Can you work these out from the model? Positions are in its coordinate system, mm. Face numbers are marked on the shaded views. A direction names the side the tool comes from. Coordinates: 2 decimals unless noted, no trailing zeros. Order: outer loops, then holes, each group sorted by start corner. A loop starts at its lowest first (then second) coordinate and runs counter-clockwise, first axis right, second up. Notation, with made-up numbers: M 67.25,86.5 L 90.25,86.5 A24 ccw 90.25,117.5 Z; hole C -40,65.5 d11. An arc over 180 degrees is marked long. Answer as CSV lines item,"result". Start each with the question number.
1. Will these pins go through, and if not, where does the flat tip stop? pin 1 (5 mm diameter, centred on y = -106.5, z = 1257.5, fed in from -X); pin 2 (8 mm diameter, centred on x = 134.5, z = 938.5, fed in from -Y); pin 3 (10 mm diameter, centred on y = -179, z = 1516.5, fed in from +X).
2. If we section it at A-A (x = 239): List the corners of the cut face in (y, z) for me.
3. I need wall thicknesses on line 1 along Z through (x, y) = (267, -102.5); line 2 along X through (y, z) = (-146, 1263.5). Which ranges of each line are inside material? Lowest first, please. Write a range as from..to.
4. If we section it at D-D (z = 1408): List the corners of the cut face in (x, y) for me, plus the area to 3 significant figures.
5. On a 3-axis mill with a long thin cutter (end or side, diameter ignored), from which of +Z, -Z, +X, -X, +Y, -Y can I reach the whole of each face in a straight line? I mean the marked faces 1, 2 and 3. Say none if no direction works.
6. If we section it at B-B (y = 0): List the corners of the cut face in (x, z) for me.
7. If we mould it in two halves opening along Z, with no side actions, what happens to the marked faces 4, 5 and 6? For each: released by +Z, released by -Z, zero draft, split by the parting line, or undercut.
```python
from build123d import *

# Parameters (mm, degrees)
F1_START = 1850
F0_R     = 300
F0_W     = 400
F0_H     = 400
F1_DEPTH = 20
F2_DEPTH = 1850
F3_DEPTH = 50


with BuildPart() as f1:
    # F0 (on Top) → F1 (new body)
    with BuildSketch(Plane.XY.offset(F1_START)):
        Circle(F0_R)
        Rectangle(F0_W, F0_H, mode=Mode.SUBTRACT)
        Rectangle(F0_W, F0_H)
    extrude(amount=F1_DEPTH)

    # F0 (on Top) → F2 (join)
    with BuildSketch(Plane.XY):
        Rectangle(F0_W, F0_H)
    extrude(amount=F2_DEPTH)

    # F0 (on Top) → F3 (join)
    with BuildSketch(Plane.XY):
        Circle(F0_R)
        Rectangle(F0_W, F0_H, mode=Mode.SUBTRACT)
    extrude(amount=F3_DEPTH)


solid = f1.part
```
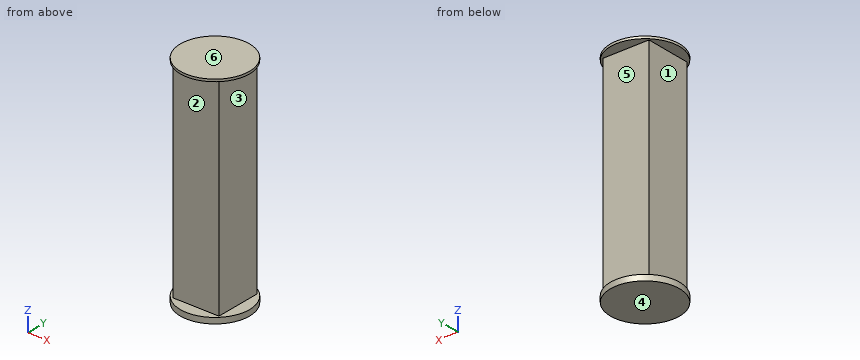
Solved:
1,pin 1,"x = -200"
1,pin 2,"y = -200"
1,pin 3,"x = 200"
2,outline,"M -181.33,0 L 181.33,0 L 181.33,50 L -181.33,50 Z; M -181.33,1850 L 181.33,1850 L 181.33,1870 L -181.33,1870 Z"
3,line 1,"0..50, 1850..1870"
3,line 2,"-200..200"
4,outline,"M -200,-200 L 200,-200 L 200,200 L -200,200 Z"
4,area,"160,000 mm²"
5,face 1,"-X, +Y, -Y"
5,face 2,"+X, -X, -Y"
5,face 3,"+X, +Y, -Y"
6,outline,"M -300,0 L 300,0 L 300,50 L 200,50 L 200,1850 L 300,1850 L 300,1870 L -300,1870 L -300,1850 L -200,1850 L -200,50 L -300,50 Z"
7,face 4,"released by -Z"
7,face 5,"undercut"
7,face 6,"released by +Z"
